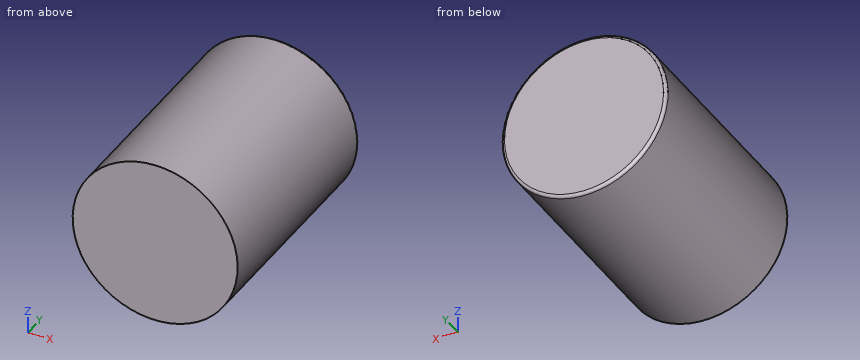
```python
from build123d import *

# Parameters (mm, degrees)
SKETCH2_R          = 29.716008705
CUT_EXTRUDE1_DEPTH = 3
FILLET1_R          = 1


with BuildPart() as part:
    # Sketch1 → Revolve1 (revolve)
    with BuildSketch(Plane.XY, mode=Mode.PRIVATE) as revolve1_sk:
        Polygon((543.090410183, 122.80292457), (571.090410183, 122.80292457), (571.090410183, 43.204678726), (552.249882464, 43.204678726), (546.251643979, 44.096308771), (543.090410183, 45.879568862), align=None)
    revolve(revolve1_sk.sketch.rotate(Axis((571.090410183, 122.80292457, 0), (0, -1, 0)), 270), axis=Axis((571.090410183, 122.80292457, 0), (0, -1, 0)))

    # Sketch2 → Cut-Extrude1 (cut)
    with BuildSketch(Plane(origin=(0, 43.204678726, 0), x_dir=(-1, 0, 0), z_dir=(0, -1, 0))):
        with Locations((-571.090410183, 0)):
            Circle(SKETCH2_R)
    extrude(amount=-CUT_EXTRUDE1_DEPTH, mode=Mode.SUBTRACT)

    # Fillet1
    fillet1_edges = [part.edges().sort_by_distance(p)[0] for p in [
        (571.090410183, 122.80292457, -28),
    ]]
    fillet(fillet1_edges, radius=FILLET1_R)


solid = part.part
```
Geometry: final body of the model. Coordinates: model frame, mm. Coordinates: 2 decimals unless noted, no trailing zeros. Loops run counter-clockwise (first coordinate to the right, second up) from the corner with the lowest first, then second, coordinate; pieces in that order, holes last. Notation, with made-up numbers: (55, 15.5) -> (96, 15.5) arc R19 cw to (96, 52.5) -> close; hole circle Ø9 at (67, 80). An arc over 180 degrees is marked (long way). Use a Markdown table: item, result. Add a question column.
(1) Pin query (flat end, axial travel): pin 1 Ø8 at (x, y) = (555, 64.5) entering from -Z; pin 2 Ø10 at (y, z) = (100.5, 1.5) entering from -X; pin 3 Ø4 at (x, y) = (568, 88.5) entering from -Z. Return the tip coordinate at first contact, or that it passes through.
(2) Line query: line 1 along X through (y, z) = (85, -1); line 2 along X through (y, z) = (98.5, 5); line 3 along Z through (x, y) = (557.5, 88). Output: solid intervals per line, ascending.
(3) Section query A-A, the plane y = 76. Return loops of the section in (x, z), plus the area to 3 significant figures.
Answer:
| question | item | result |
|---|---|---|
| 1 | pin 1 | stops at z = -25.26 |
| 1 | pin 2 | stops at x = 543.09 |
| 1 | pin 3 | stops at z = -27.98 |
| 2 | line 1 | x = 543.11 to 599.07 |
| 2 | line 2 | x = 543.54 to 598.64 |
| 2 | line 3 | z = -24.48 to 24.48 |
| 3 | outline | circle Ø56 at (571.09, 0) |
| 3 | area | 2,460 mm^2 |
